The drawing under review shows one solid part. Ordinate dimensions are in mm from its lowest x, y, z. Give positions to 0.01 mm unless a question says otherwise; leave off trailing zeros. Write each loop counter-clockwise with the first axis right and the second up, starting at its lowest first coordinate (ties: lowest second). Pieces come first, ordered by that corner, then holes.
Q1. We need section D-D (y = 26.25). Write out the cut boundary in (x, z).
Q2. For line 1 (X direction, y = 17.75, z = 0.4); line 2 (Y direction, x = 10.5, z = 0.3); line 3 (X direction, y = 25.25, z = 0.65), list the stretches that pass through material, from the lowest coordinate up.
Q3. We need section C-C (x = 53.5). Write out the cut boundary in (y, z).
Q4. We need section A-A (y = 18). Write out the cut boundary in (x, z), then the cut area to 3 significant figures.
Q5. We need section B-B (z = 1.55). Write out the cut boundary in (x, y), then the cut area to 3 significant figures.
Q6. Insertion check: P1, Ø7, axis at x = 52, y = 18, coming from the +Z side; P2, Ø1.5, axis at x = 25.5, z = 1.5, coming from the +Y side. Each pin has a flat end and moves straight along its axis. Give the tip position at first contact, or say it passes through.
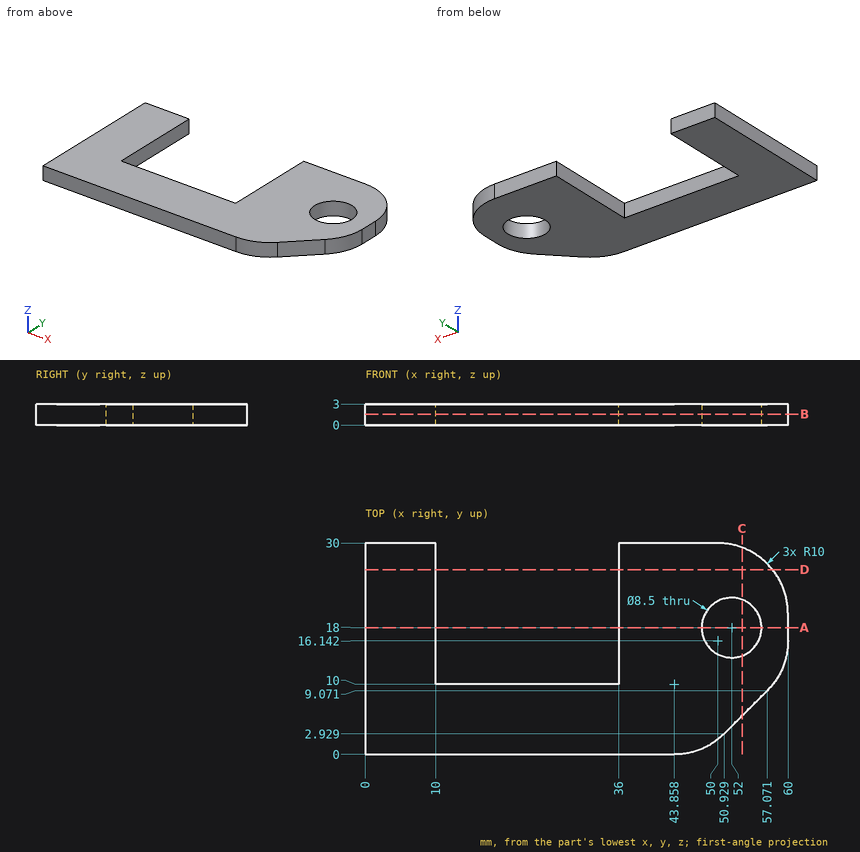
Computed:
1. outline: (0, 0) - (10, 0) - (10, 3) - (0, 3) - close; (36, 0) - (57.81, 0) - (57.81, 3) - (36, 3) - close
2. line 1: x = 0 to 10, 36 to 47.76, 56.24 to 60
2. line 2: y = 0 to 10
2. line 3: x = 0 to 10, 36 to 58.51
3. outline: (5.5, 0) - (14.02, 0) - (14.02, 3) - (5.5, 3) - close; (21.98, 0) - (29.37, 0) - (29.37, 3) - (21.98, 3) - close
4. outline: (0, 0) - (10, 0) - (10, 3) - (0, 3) - close; (36, 0) - (47.75, 0) - (47.75, 3) - (36, 3) - close; (56.25, 0) - (60, 0) - (60, 3) - (56.25, 3) - close
4. area: 76.5 mm2
5. outline: (0, 0) - (43.86, 0) arc R10 ccw to (50.93, 2.93) - (57.07, 9.07) arc R10 ccw to (60, 16.14) - (60, 20) arc R10 ccw to (50, 30) - (36, 30) - (36, 10) - (10, 10) - (10, 30) - (0, 30) - close; hole circle Ø8.5 at (52, 18)
5. area: 1,130 mm2
6. P1: passes through
6. P2: stops at y = 10
